Check sheet for the modelled part. Datum: model origin and axes. Units: mm. A direction names the side the tool comes from. Give positions to 0.01 mm unless a question says otherwise; leave off trailing zeros. Order: outer loops, then holes, each group sorted by start corner. A loop starts at its lowest first (then second) coordinate and runs counter-clockwise, first axis right, second up.
Item 1: Sectioned sample at C-C on y = 3.25. Record the boundary of the cut face in (x, z), and give its area (3 significant figures).
Item 2: Sectioned sample at B-B on z = 8.75. Record the boundary of the cut face in (x, y).
Item 3: Access from +Z, -Z, +X, -X, +Y, -Y to the whole of each face (thin tool, end or side, straight path). Record for faces 1 (the cylindrical face through (-8.2, 0.76, -3.03)), 2 (the cylindrical face through (-7.305, 2.768, -6.874)).
Item 4: Material ranges on line 1 along X through (y, z) = (3.5, 5); line 2 along Y through (x, z) = (-1.25, -2.25); line 3 along X through (y, z) = (2.5, -6.5), recorded low to high.
Item 5: Sectioned sample at D-D on z = 3.25. Record the boundary of the cut face in (x, y), and give its area (3 significant figures).
Item 6: Release check for a two-part mould opening along X. For faces 3 (the flat face through (3, 0, 3)), 4 (the cylindrical face through (1.561, 2.768, 5.555)), 5 (the cylindrical face through (-14.985, 1.972, -0.66)), 6 (the cylindrical face through (4.627, 2.768, -2.236)) record: released by +X, released by -X, zero draft, split by the parting line, or undercut.
Item 7: Gauge pin test, flat ends, axial feed: P1, Ø5, axis at x = 6.93, z = 4, coming from the +Y side; P2, Ø4.5, axis at x = -8.5, z = -5, coming from the +Y side; P3, Ø1.5, axis at x = -4, y = 4, coming from the +Z side; P4, Ø2.5, axis at x = -6.93, z = 4, coming from the +Y side. Record the tip position at first contact, or that the pin passes through.
Item 8: Sectioned sample at A-A on x = 0. Record the boundary of the cut face in (y, z), and give its area (3 significant figures).
from build123d import *

# Parameters (mm, degrees)
SKETCH_1_R          = 15
EXTRUDE_1_DEPTH     = 4
SKETCH_2_R          = 1.6
CUT_EXTRUDE_1_DEPTH = 5
SKETCH_3_R          = 2.9
CUT_EXTRUDE_2_DEPTH = 2.5
SKETCH_4_R          = 5
EXTRUDE_2_DEPTH     = 18
SKETCH_5_R          = 4
CUT_EXTRUDE_3_DEPTH = 2


with BuildPart() as part:
    # 草图1 → 凸台-拉伸1 (new body)
    with BuildSketch(Plane(origin=(0, 0, 0), x_dir=(1, 0, 0), z_dir=(0, 1, 0))):
        Circle(SKETCH_1_R)
    extrude(amount=EXTRUDE_1_DEPTH)

    # 草图2 → 切除-拉伸1 (cut)
    with BuildSketch(Plane(origin=(0, 4, 0), x_dir=(1, 0, 0), z_dir=(0, 1, 0))):
        with Locations((0, 8)):
            Circle(SKETCH_2_R)
        with Locations((6.92820323, 4)):
            Circle(SKETCH_2_R)
        with Locations((6.92820323, -4)):
            Circle(SKETCH_2_R)
        with Locations((0, -8)):
            Circle(SKETCH_2_R)
        with Locations((-6.92820323, -4)):
            Circle(SKETCH_2_R)
        with Locations((-6.92820323, 4)):
            Circle(SKETCH_2_R)
    extrude(amount=-CUT_EXTRUDE_1_DEPTH, mode=Mode.SUBTRACT)

    # 草图3 → 切除-拉伸2 (cut)
    with BuildSketch(Plane(origin=(0, 4, 0), x_dir=(1, 0, 0), z_dir=(0, 1, 0))):
        with Locations((0, 8)):
            Circle(SKETCH_3_R)
        with Locations((6.92870323, 4.000866025)):
            Circle(SKETCH_3_R)
        with Locations((6.92970323, -3.999133975)):
            Circle(SKETCH_3_R)
        with Locations((0.002, -8)):
            Circle(SKETCH_3_R)
        with Locations((-6.92670323, -4.000866025)):
            Circle(SKETCH_3_R)
        with Locations((-6.92770323, 3.999133975)):
            Circle(SKETCH_3_R)
    extrude(amount=-CUT_EXTRUDE_2_DEPTH, mode=Mode.SUBTRACT)

    # 草图4 → 凸台-拉伸2 (add)
    with BuildSketch(Plane(origin=(0, 4, 0), x_dir=(1, 0, 0), z_dir=(0, 1, 0))):
        Circle(SKETCH_4_R)
    extrude(amount=EXTRUDE_2_DEPTH)

    # 草图5 → 切除-拉伸3 (cut)
    with BuildSketch(Plane.XZ):
        Circle(SKETCH_5_R)
    extrude(amount=-CUT_EXTRUDE_3_DEPTH, mode=Mode.SUBTRACT)


solid = part.part
Report:
1. outline: circle Ø30 at (0, 0); hole circle Ø5.8 at (-6.93, -4); hole circle Ø5.8 at (-6.93, 4); hole circle Ø5.8 at (0, -8); hole circle Ø5.8 at (0, 8); hole circle Ø5.8 at (6.93, -4); hole circle Ø5.8 at (6.93, 4)
1. area: 548 mm2
2. outline: (-12.18, 0) - (-1.41, 0) - (-1.41, 1.5) - (-2.8, 1.5) - (-2.8, 4) - (-12.18, 4) - close; (1.41, 0) - (12.18, 0) - (12.18, 4) - (2.8, 4) - (2.8, 1.5) - (1.41, 1.5) - close
3. face 1: +Y, -Y
3. face 2: +Y
4. line 1: x = -14.14 to -9.65, -4.2 to 4.21, 9.65 to 14.14
4. line 2: y = 2 to 22
4. line 3: x = -13.52 to -8.4, -5.46 to -2.48, 2.48 to 5.46, 8.4 to 13.52
5. outline: (-14.64, 0) - (-8.34, 0) - (-8.34, 1.5) - (-9.73, 1.5) - (-9.73, 4) - (-14.64, 4) - close; (-5.51, 0) - (-2.33, 0) - (-2.33, 2) - (2.33, 2) - (2.33, 0) - (5.51, 0) - (5.51, 1.5) - (4.13, 1.5) - (4.13, 4) - (3.8, 4) - (3.8, 22) - (-3.8, 22) - (-3.8, 4) - (-4.13, 4) - (-4.13, 1.5) - (-5.51, 1.5) - close; (8.34, 0) - (14.64, 0) - (14.64, 4) - (9.73, 4) - (9.73, 1.5) - (8.34, 1.5) - close
5. area: 208 mm2
6. face 3: zero draft
6. face 4: undercut
6. face 5: split by the parting line
6. face 6: undercut
7. P1: stops at y = 1.5
7. P2: stops at y = 4
7. P3: stops at z = 14.64
7. P4: passes through
8. outline: (0, -15) - (4, -15) - (4, -10.9) - (1.5, -10.9) - (1.5, -9.6) - (0, -9.6) - close; (0, -6.4) - (1.5, -6.4) - (1.5, -5.1) - (4, -5.1) - (4, -5) - (22, -5) - (22, 5) - (4, 5) - (4, 5.1) - (1.5, 5.1) - (1.5, 6.4) - (0, 6.4) - (0, 4) - (2, 4) - (2, -4) - (0, -4) - close; (0, 9.6) - (1.5, 9.6) - (1.5, 10.9) - (4, 10.9) - (4, 15) - (0, 15) - close
8. area: 245 mm2
